```python
from build123d import *

# Parameters (mm, degrees)
F1_DEPTH = 50
F3_D     = 2.4
F5_D     = 2.4
F6_SIZE  = 2


with BuildPart() as f1:
    # F0 (on Front) → F1 (new body)
    with BuildSketch(Plane.XZ):
        Polygon((0, -40), (0, 0), (40, 0), (40, 4), (0, 8), (-8, 0), (-4, -40), align=None)
    extrude(amount=F1_DEPTH)

    # F3 (through all)
    with Locations(Plane(origin=(0, 0, 0), x_dir=(1, 0, 0), z_dir=(0, 0, -1))):
        with Locations((32, 42), (32, 8), (7, 8), (7, 42)):
            Hole(F3_D / 2)

    # F5 (through all)
    with Locations(Plane.YZ):
        with Locations((-42, -32), (-42, -14), (-8, -32), (-8, -14)):
            Hole(F5_D / 2)

    # F6
    f6_edges = [f1.edges().sort_by_distance(p)[0] for p in [
        (20, -50, 6),
        (-4, -50, 4),
        (-6, -50, -20),
        (-6, 0, -20),
        (20, 0, 6),
        (-4, 0, 4),
    ]]
    chamfer(f6_edges, length=F6_SIZE)


solid = f1.part
```
Geometry check sheet. Reference: the model listing, model coordinates, mm. Coordinates: 2 decimals unless noted, no trailing zeros. Loops run counter-clockwise (first coordinate to the right, second up) from the corner with the lowest first, then second, coordinate; pieces in that order, holes last.
Item 1: Thickness scan on line 1 (Y direction, x = 7, z = 3.75); line 2 (X direction, y = -42, z = 3.35); line 3 (X direction, y = -42, z = 2.9). Record the ranges inside material, lowest first.
Item 2: Sectioned sample at C-C, the plane z = -14. Record the boundary of the cut face in (x, y), then the cut area to 3 significant figures.
Item 3: Sectioned sample at A-A, the plane y = -42. Record the boundary of the cut face in (x, z), then the cut area to 3 significant figures.
Item 4: Release check for a two-part mould opening along Y. For faces 1 (the face through (30.855, -42.36, 2.494)), 2 (the face through (-5.037, -48.986, -19.72)), 3 (the face through (-3.247, -1.014, 3.359)) record: released by +Y, released by -Y, zero draft, split by the parting line, or undercut.
Item 5: Sectioned sample at D-D, the plane z = -34. Record the boundary of the cut face in (x, y).
Item 6: Go/stop test with flat-tipped pins: pin 1 Ø5 at (x, y) = (19.5, -13) entering from +Z; pin 2 Ø3 at (x, y) = (7, -42) entering from +Z; pin 3 Ø12 at (y, z) = (-14.5, -31) entering from -X. Record where each tip stops, or that it passes through.
Item 7: Sectioned sample at B-B, the plane x = 7. Record the boundary of the cut face in (y, z), then the cut area to 3 significant figures.
Check result:
1. line 1: y = -50 to -43.2, -40.8 to -9.2, -6.8 to 0
1. line 2: x = -4.65 to 5.8, 8.2 to 30.8, 33.2 to 40
1. line 3: x = -5.1 to 5.8, 8.2 to 30.8, 33.2 to 40
2. outline: (-6.6, -48) - (-4.59, -50) - (0, -50) - (0, -43.2) - (-6.6, -43.2) - close; (-6.6, -40.8) - (0, -40.8) - (0, -9.2) - (-6.6, -9.2) - close; (-6.6, -6.8) - (0, -6.8) - (0, 0) - (-4.59, 0) - (-6.6, -2) - close
2. area: 294 mm2
3. outline: (-8, 0) - (-6.72, -12.8) - (0, -12.8) - (0, 0) - (5.8, 0) - (5.8, 7.42) - (0, 8) - close; (-6.48, -15.2) - (-4.92, -30.8) - (0, -30.8) - (0, -15.2) - close; (-4.68, -33.2) - (-4, -40) - (0, -40) - (0, -33.2) - close; (8.2, 0) - (30.8, 0) - (30.8, 4.92) - (8.2, 7.18) - close; (33.2, 0) - (40, 0) - (40, 4) - (33.2, 4.68) - close
3. area: 456 mm2
4. face 1: undercut
4. face 2: released by -Y
4. face 3: released by +Y
5. outline: (-4.6, -48) - (-2.59, -50) - (0, -50) - (0, 0) - (-2.59, 0) - (-4.6, -2) - close
6. pin 1: stops at z = 6.3
6. pin 2: stops at z = 7.45
6. pin 3: stops at x = -5.5
7. outline: (-50, 0) - (-43.2, 0) - (-43.2, 7.3) - (-48, 7.3) - (-50, 5.29) - close; (-40.8, 0) - (-9.2, 0) - (-9.2, 7.3) - (-40.8, 7.3) - close; (-6.8, 0) - (0, 0) - (0, 5.29) - (-2, 7.3) - (-6.8, 7.3) - close
7. area: 326 mm2
